from build123d import *

# Parameters (mm, degrees)
F0_R     = 20.37
F0_R_2   = 6.4
F1_DEPTH = 1.2
F2_DEPTH = 5.7
F3_R     = 0.3


with BuildPart() as f1:
    # F0 (on Top) → F1 (new body)
    with BuildSketch(Plane.XY):
        Circle(F0_R)
        Circle(F0_R_2, mode=Mode.SUBTRACT)
        Circle(F0_R_2)
        with BuildLine():
            ThreePointArc((-1.2, 1.2041594579), (1.7, 0), (-1.2, -1.2041594579))
            Line((-1.2, -1.2041594579), (-1.2, 1.2041594579))
        make_face(mode=Mode.SUBTRACT)
        with BuildLine():
            Line((-1.2, 1.2041594579), (-1.2, -1.2041594579))
            ThreePointArc((-1.2, -1.2041594579), (1.7, 0), (-1.2, 1.2041594579))
        make_face()
    extrude(amount=-F1_DEPTH)

    # F0 (on Top) → F2 (join)
    with BuildSketch(Plane.XY):
        Circle(F0_R_2)
        with BuildLine():
            ThreePointArc((-1.2, 1.2041594579), (1.7, 0), (-1.2, -1.2041594579))
            Line((-1.2, -1.2041594579), (-1.2, 1.2041594579))
        make_face(mode=Mode.SUBTRACT)
    extrude(amount=F2_DEPTH)

    # F3
    f3_edges = [f1.edges().sort_by_distance(p)[0] for p in [
        (-20.37, 0, -1.2),
        (-6.4, 0, 5.7),
    ]]
    fillet(f3_edges, radius=F3_R)


solid = f1.part
Build history of the part. All positions in model axes, mm. A direction names the side the tool comes from. Round coordinates to 2 decimals unless told otherwise and drop trailing zeros. Write each loop counter-clockwise with the first axis right and the second up, starting at its lowest first coordinate (ties: lowest second). Pieces come first, ordered by that corner, then holes. Notation, with made-up numbers: (-10, 82.5) -> (40, 82.5) arc R18 ccw to (40, 109.5) -> close; hole circle Ø7 at (34.25, 4.5). An arc over 180 degrees is marked (long way). Write item = value, one per line.
(1) Tool access for faces 5 (the face through (0, 0, -1.2)), 6 (the face through (-1.2, 0, 3)): list every direction of +Z, -Z, +X, -X, +Y, -Y with a clear straight run to the whole face (end or side of a thin tool).
Answer:
face_5 = -Z, +X, -X, +Y, -Y
face_6 = +Z
(2) Band-saw the part on A-A (x = 0). Give the cut face in (y, z).
Answer:
outline = (-20.37, -0.9) arc R0.3 ccw to (-20.07, -1.2) -> (20.07, -1.2) arc R0.3 ccw to (20.37, -0.9) -> (20.37, 0) -> (6.4, 0) -> (6.4, 5.4) arc R0.3 ccw to (6.1, 5.7) -> (1.7, 5.7) -> (1.7, 0) -> (-1.7, 0) -> (-1.7, 5.7) -> (-6.1, 5.7) arc R0.3 ccw to (-6.4, 5.4) -> (-6.4, 0) -> (-20.37, 0) -> close
(3) Probe L1, parallel to Y at x = 0, z = 2.4; L2, parallel to Z at x = -1, y = 11; L3, parallel to X at y = 2.5, z = 4.5. List the from-to ranges inside material, lowest first.
Answer:
L1 = -6.4 to -1.7, 1.7 to 6.4
L2 = -1.2 to 0
L3 = -5.89 to 5.89
(4) Flat gauge pins, fed straight in: pin 1 (1.9 mm diameter, centred on y = 0, z = 2, fed in from +X); pin 2 (12 mm diameter, centred on x = 0.5, y = 15, fed in from +Z). Where does each tip first touch, or does it go through?
Answer:
pin_1 = 6.4
pin_2 = 0
(5) Two-plate mould, pull along Y, no slides. Class faces 1 (the face through (10.951, 17.176, -0.444)), 2 (the face through (0, 0, 0)), 3 (the face through (-1.4, 0.1, 5.7)), 4 (the face through (1.7, 0.06, 2.81)): pulls with the +Y half, pulls with the -Y half, needs draft (parallel to the pull), parting line crosses it, or undercut.
Answer:
face_1 = parting line crosses it
face_2 = undercut
face_3 = needs draft
face_4 = undercut
(6) Band-saw the part on C-C (z = 0.75). Give the cut face in (x, y), then the cut area to 3 significant figures.
Answer:
outline = circle Ø12.8 at (0, 0); hole (-1.2, -1.2) arc R1.7 ccw (long way) to (-1.2, 1.2) -> close
area = 120 mm2
(7) Band-saw the part on B-B (y = 0). Give the cut face in (x, z), then the cut area to 3 significant figures.
Answer:
outline = (-20.37, -0.9) arc R0.3 ccw to (-20.07, -1.2) -> (20.07, -1.2) arc R0.3 ccw to (20.37, -0.9) -> (20.37, 0) -> (6.4, 0) -> (6.4, 5.4) arc R0.3 ccw to (6.1, 5.7) -> (1.7, 5.7) -> (1.7, 0) -> (-1.2, 0) -> (-1.2, 5.7) -> (-6.1, 5.7) arc R0.3 ccw to (-6.4, 5.4) -> (-6.4, 0) -> (-20.37, 0) -> close
area = 105 mm2
